Here's how the part is built. I have some questions about the finished solid (model axes, mm). Face numbers are marked on the shaded views. A direction names the side the tool comes from. Coordinates: 2 decimals unless noted, no trailing zeros. Write each loop counter-clockwise with the first axis right and the second up, starting at its lowest first coordinate (ties: lowest second). Pieces come first, ordered by that corner, then holes. Notation, with made-up numbers: (8, 53.25) -> (26, 53.25) arc R9 cw to (26, 63.25) -> close; hole circle Ø9 at (-35, 17.25). An arc over 180 degrees is marked (long way). Use a Markdown table: item, result. Add a question column.
Item 1: Will these pins go through, and if not, where does the flat tip stop? pin 1 Ø4.5 at (y, z) = (-17, -6) entering from -X; pin 2 Ø1.8 at (x, z) = (-5, -5) entering from -Y (3 decimals); pin 3 Ø10 at (y, z) = (-22, 43.5) entering from -X; pin 4 Ø1.9 at (x, z) = (-15.24, -3.81) entering from -Y (3 decimals).
Item 2: If we mould it in two halves opening along X, with no side actions, what happens to the marked faces 1, 2 and 3? For each: pulls with the +X half, pulls with the -X half, needs draft (parallel to the pull), parting line crosses it, or undercut.
Item 3: Imagine slicing it at C-C, the plane x = -21.5. Write out the boundary of the cut face in (y, z) (3 decimals).
Item 4: Imagine slicing it at A-A, the plane z = 13.5. Write out the boundary of the cut face in (x, y) (3 decimals).
Item 5: Imagine slicing it at B-B, the plane x = -10.16. Write out the boundary of the cut face in (y, z) (3 decimals).
Item 6: If I drill on line 1 along Z through (x, y) = (-5, -1) (3 decimals); line 2 along Z through (x, y) = (-13, -2.5) (3 decimals); line 3 along X through (y, z) = (-19, 16) (3 decimals), over which ranges is the centre line in solid material (lowest first)? Write a range as from..to.
Item 7: On a 3-axis mill with a long thin cutter (end or side, diameter ignored), from which of +Z, -Z, +X, -X, +Y, -Y can I reach the whole of each face in a straight line? I mean the marked faces 4, 5, 6, 7 and 8. Say none if no direction works.
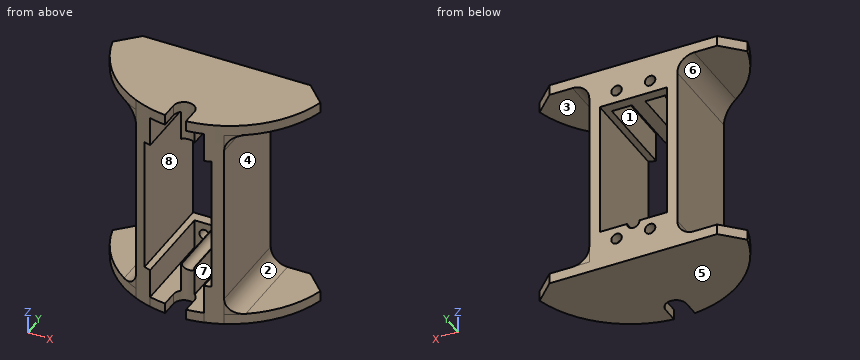
```python
from build123d import *

# Parameters (mm, degrees)
F0_W          = 26.67
F0_H          = 58.928
F0_R          = 1.5875
F1_DEPTH      = 3.175
F2_W          = 4.064
F2_H          = 8.89
F3_DEPTH      = 38.1
F5_DEPTH      = 101.6
F7_DEPTH      = 3.175
F9_DEPTH      = 3.175
F11_DEPTH     = 127
F12_T4_DEPTH  = 40.3062822545
F12_S5_R      = 32.5
F12_T6_DEPTH  = 22
F12_T10_DEPTH = 40.3062822545
F12_S11_R     = 32.5
F12_T12_DEPTH = 22
F12_T16_DEPTH = 40.3062822545
F12_S17_R     = 32.5
F12_T18_DEPTH = 22
F12_T22_DEPTH = 40.3062822545
F12_S23_R     = 32.5
F12_T24_DEPTH = 22


# Not quite as in the source:
# - a fillet or chamfer that OpenCascade refuses, or shapes differently, is made with other operations: its cross-section is extruded or revolved along the edge and cut away or added
# - after a boolean that leaves OpenCascade's solid faulty, fix() repairs it


with BuildPart() as f1:
    # F0 (on Front) → F1 (new body)
    with BuildSketch(Plane.XZ):
        with Locations((-10.16, 20.574)):
            Rectangle(F0_W, F0_H)
        with Locations((-15.24, -3.81)):
            Circle(F0_R, mode=Mode.SUBTRACT)
        with BuildLine():
            Line((0, 41.148), (0, 0))
            Line((0, 0), (-8.255, 0))
            ThreePointArc((-8.255, 0), (-10.16, -1.905), (-12.065, 0))
            Line((-12.065, 0), (-20.32, 0))
            Line((-20.32, 0), (-20.32, 41.148))
            Line((-20.32, 41.148), (0, 41.148))
        make_face(mode=Mode.SUBTRACT)
        with Locations((-5.08, -3.81)):
            Circle(F0_R, mode=Mode.SUBTRACT)
        with Locations((-15.24, 44.958)):
            Circle(F0_R, mode=Mode.SUBTRACT)
        with Locations((-5.08, 44.958)):
            Circle(F0_R, mode=Mode.SUBTRACT)
    extrude(amount=F1_DEPTH)

    # F2 (on face) → F3 (join)
    with BuildSketch(Plane.XZ.offset(3.175)):
        Polygon((0, 0), (-2.032, 0), (-2.032, -8.89), (3.175, -8.89), (3.175, 50.038), (-2.032, 50.038), (-2.032, 41.148), (0, 41.148), align=None)
        with BuildLine():
            Line((-8.128, -8.89), (-8.128, 0))
            Line((-8.128, 0), (-8.255, 0))
            ThreePointArc((-8.255, 0), (-10.16, -1.905), (-12.065, 0))
            Line((-12.065, 0), (-12.192, 0))
            Line((-12.192, 0), (-12.192, -8.89))
            Line((-12.192, -8.89), (-8.128, -8.89))
        make_face()
        Polygon((-23.495, -8.89), (-18.288, -8.89), (-18.288, 0), (-20.32, 0), (-20.32, 41.148), (-18.288, 41.148), (-18.288, 50.038), (-23.495, 50.038), align=None)
        with Locations((-10.16, 45.593)):
            Rectangle(F2_W, F2_H)
    extrude(amount=F3_DEPTH)

    # F4 (on face) → F5 (intersect)
    with BuildSketch(Plane.XY.offset(50.038)):
        with BuildLine():
            Line((-23.495, 0), (-23.495, -27.6062822545))
            ThreePointArc((-23.495, -27.6062822545), (-20.9303918657, -28.6314743475), (-18.288, -29.4352149387))
            Line((-18.288, -29.4352149387), (-18.288, -3.175))
            Line((-18.288, -3.175), (-12.192, -3.175))
            Line((-12.192, -3.175), (-12.192, -30.4044143518))
            ThreePointArc((-12.192, -30.4044143518), (-10.16, -30.468), (-8.128, -30.4044143518))
            Line((-8.128, -30.4044143518), (-8.128, -3.175))
            Line((-8.128, -3.175), (-2.032, -3.175))
            Line((-2.032, -3.175), (-2.032, -29.4352149387))
            ThreePointArc((-2.032, -29.4352149387), (0.6103918657, -28.6314743475), (3.175, -27.6062822545))
            Line((3.175, -27.6062822545), (3.175, 0))
            Line((3.175, 0), (-10.16, 0))
            Line((-10.16, 0), (-23.495, 0))
        make_face()
    extrude(amount=-F5_DEPTH, mode=Mode.INTERSECT)

    # F6 (on face) → F7 (join)
    with BuildSketch(Plane(origin=(0, 0, -8.89), x_dir=(1, 0, 0), z_dir=(0, 0, -1))):
        with BuildLine():
            Line((15.24, 0), (21.313116807, 6.073116807))
            ThreePointArc((21.313116807, 6.073116807), (14.6968126777, 18.9057377838), (3.175, 27.6062822545))
            Line((3.175, 27.6062822545), (3.175, 0))
            Line((3.175, 0), (15.24, 0))
        make_face()
        with BuildLine():
            Line((3.175, 0), (3.175, 27.6062822545))
            ThreePointArc((3.175, 27.6062822545), (0.6103918657, 28.6314743475), (-2.032, 29.4352149387))
            Line((-2.032, 29.4352149387), (-2.032, 3.175))
            Line((-2.032, 3.175), (-8.128, 3.175))
            Line((-8.128, 3.175), (-8.128, 30.4044143518))
            ThreePointArc((-8.128, 30.4044143518), (-10.16, 30.468), (-12.192, 30.4044143518))
            Line((-12.192, 30.4044143518), (-12.192, 3.175))
            Line((-12.192, 3.175), (-18.288, 3.175))
            Line((-18.288, 3.175), (-18.288, 29.4352149387))
            ThreePointArc((-18.288, 29.4352149387), (-20.9303918657, 28.6314743475), (-23.495, 27.6062822545))
            Line((-23.495, 27.6062822545), (-23.495, 0))
            Line((-23.495, 0), (-10.16, 0))
            Line((-10.16, 0), (3.175, 0))
        make_face()
        with BuildLine():
            Line((-2.032, 3.175), (-2.032, 29.4352149387))
            ThreePointArc((-2.032, 29.4352149387), (-5.0569384801, 30.0648653162), (-8.128, 30.4044143518))
            Line((-8.128, 30.4044143518), (-8.128, 3.175))
            Line((-8.128, 3.175), (-2.032, 3.175))
        make_face()
        with BuildLine():
            Line((-12.192, 3.175), (-12.192, 30.4044143518))
            ThreePointArc((-12.192, 30.4044143518), (-15.2630615199, 30.0648653162), (-18.288, 29.4352149387))
            Line((-18.288, 29.4352149387), (-18.288, 3.175))
            Line((-18.288, 3.175), (-12.192, 3.175))
        make_face()
        with BuildLine():
            Line((-35.56, 0), (-23.495, 0))
            Line((-23.495, 0), (-23.495, 27.6062822545))
            ThreePointArc((-23.495, 27.6062822545), (-35.0168126777, 18.9057377838), (-41.633116807, 6.073116807))
            Line((-41.633116807, 6.073116807), (-35.56, 0))
        make_face()
    extrude(amount=F7_DEPTH)

    add(f1.part.fix(), mode=Mode.REPLACE)

    # F8 (on face) → F9 (join)
    with BuildSketch(Plane.XY.offset(50.038)):
        with BuildLine():
            Line((-23.495, -27.6062822545), (-23.495, 0))
            Line((-23.495, 0), (-35.56, 0))
            Line((-35.56, 0), (-41.633116807, -6.073116807))
            ThreePointArc((-41.633116807, -6.073116807), (-35.0168126777, -18.9057377838), (-23.495, -27.6062822545))
        make_face()
        with BuildLine():
            Line((15.24, 0), (3.175, 0))
            Line((3.175, 0), (3.175, -27.6062822545))
            ThreePointArc((3.175, -27.6062822545), (14.6968126777, -18.9057377838), (21.313116807, -6.073116807))
            Line((21.313116807, -6.073116807), (15.24, 0))
        make_face()
        with BuildLine():
            Line((-18.288, -3.175), (-18.288, -29.4352149387))
            ThreePointArc((-18.288, -29.4352149387), (-15.2630615199, -30.0648653162), (-12.192, -30.4044143518))
            Line((-12.192, -30.4044143518), (-12.192, -3.175))
            Line((-12.192, -3.175), (-18.288, -3.175))
        make_face()
        with BuildLine():
            ThreePointArc((-8.128, -30.4044143518), (-5.0569384801, -30.0648653162), (-2.032, -29.4352149387))
            Line((-2.032, -29.4352149387), (-2.032, -3.175))
            Line((-2.032, -3.175), (-8.128, -3.175))
            Line((-8.128, -3.175), (-8.128, -30.4044143518))
        make_face()
        with BuildLine():
            Line((3.175, -27.6062822545), (3.175, 0))
            Line((3.175, 0), (-23.495, 0))
            Line((-23.495, 0), (-23.495, -27.6062822545))
            ThreePointArc((-23.495, -27.6062822545), (-20.9303918657, -28.6314743475), (-18.288, -29.4352149387))
            Line((-18.288, -29.4352149387), (-18.288, -3.175))
            Line((-18.288, -3.175), (-12.192, -3.175))
            Line((-12.192, -3.175), (-12.192, -30.4044143518))
            ThreePointArc((-12.192, -30.4044143518), (-10.16, -30.468), (-8.128, -30.4044143518))
            Line((-8.128, -30.4044143518), (-8.128, -3.175))
            Line((-8.128, -3.175), (-2.032, -3.175))
            Line((-2.032, -3.175), (-2.032, -29.4352149387))
            ThreePointArc((-2.032, -29.4352149387), (0.6103918657, -28.6314743475), (3.175, -27.6062822545))
        make_face()
    extrude(amount=F9_DEPTH)

    # F10 (on face) → F11 (cut)
    with BuildSketch(Plane(origin=(0, 0, -12.065), x_dir=(1, 0, 0), z_dir=(0, 0, -1))):
        with BuildLine():
            Line((-13.335, 30.312541657), (-13.335, 25.4))
            ThreePointArc((-13.335, 25.4), (-10.16, 22.225), (-6.985, 25.4))
            Line((-6.985, 25.4), (-6.985, 30.312541657))
            ThreePointArc((-6.985, 30.312541657), (-10.16, 30.468), (-13.335, 30.312541657))
        make_face()
    extrude(amount=-F11_DEPTH, mode=Mode.SUBTRACT)

    # F12: fillet of radius 5.08 on 4 edges, made by hand


with BuildPart() as f12_tool2:
    # F12_s3 → F12_t4 (new body)
    with BuildSketch(Plane.XZ.offset(40.3062822545)):
        with BuildLine():
            ThreePointArc((-23.495, -3.81), (-24.9828975516, -7.4021024484), (-28.575, -8.89))
            Line((-28.575, -8.89), (-23.495, -8.89))
            Line((-23.495, -8.89), (-23.495, -3.81))
        make_face()
    extrude(amount=-F12_T4_DEPTH)

    # F12_s5 → F12_t6 (intersect, symmetric)
    with BuildSketch(Plane.XY.offset(-6.4)):
        with Locations((-10.16, 2.032)):
            Circle(F12_S5_R)
    extrude(amount=F12_T6_DEPTH, both=True, mode=Mode.INTERSECT)


with BuildPart() as f1_1:
    add(f1.part)

    # F12_t1: union F12_tool2
    add(f12_tool2.part)


with BuildPart() as f12_tool8:
    # F12_s9 → F12_t10 (new body)
    with BuildSketch(Plane.XZ):
        with BuildLine():
            ThreePointArc((-28.575, 50.038), (-24.9828975516, 48.5501024484), (-23.495, 44.958))
            Line((-23.495, 44.958), (-23.495, 50.038))
            Line((-23.495, 50.038), (-28.575, 50.038))
        make_face()
    extrude(amount=F12_T10_DEPTH)

    # F12_s11 → F12_t12 (intersect, symmetric)
    with BuildSketch(Plane.XY.offset(47.5)):
        with Locations((-10.16, 2.032)):
            Circle(F12_S11_R)
    extrude(amount=F12_T12_DEPTH, both=True, mode=Mode.INTERSECT)


with BuildPart() as f1_2:
    add(f1_1.part)

    # F12_t7: union F12_tool8
    add(f12_tool8.part)


with BuildPart() as f12_tool14:
    # F12_s15 → F12_t16 (new body)
    with BuildSketch(Plane.XZ):
        with BuildLine():
            ThreePointArc((3.175, 44.958), (4.6628975516, 48.5501024484), (8.255, 50.038))
            Line((8.255, 50.038), (3.175, 50.038))
            Line((3.175, 50.038), (3.175, 44.958))
        make_face()
    extrude(amount=F12_T16_DEPTH)

    # F12_s17 → F12_t18 (intersect, symmetric)
    with BuildSketch(Plane.XY.offset(47.5)):
        with Locations((-10.16, 2.032)):
            Circle(F12_S17_R)
    extrude(amount=F12_T18_DEPTH, both=True, mode=Mode.INTERSECT)


with BuildPart() as f1_3:
    add(f1_2.part)

    # F12_t13: union F12_tool14
    add(f12_tool14.part)


with BuildPart() as f12_tool20:
    # F12_s21 → F12_t22 (new body)
    with BuildSketch(Plane.XZ.offset(40.3062822545)):
        with BuildLine():
            ThreePointArc((8.255, -8.89), (4.6628975516, -7.4021024484), (3.175, -3.81))
            Line((3.175, -3.81), (3.175, -8.89))
            Line((3.175, -8.89), (8.255, -8.89))
        make_face()
    extrude(amount=-F12_T22_DEPTH)

    # F12_s23 → F12_t24 (intersect, symmetric)
    with BuildSketch(Plane.XY.offset(-6.4)):
        with Locations((-10.16, 2.032)):
            Circle(F12_S23_R)
    extrude(amount=F12_T24_DEPTH, both=True, mode=Mode.INTERSECT)


with BuildPart() as f1_4:
    add(f1_3.part)

    # F12_t19: union F12_tool20
    add(f12_tool20.part)


solid = f1_4.part
```
Ans:
| question | item | result |
|---|---|---|
| 1 | pin 1 | stops at x = -26.11 |
| 1 | pin 2 | stops at y = -3.175 |
| 1 | pin 3 | stops at x = -24.93 |
| 1 | pin 4 | passes through |
| 2 | face 1 | undercut |
| 2 | face 2 | pulls with the +X half |
| 2 | face 3 | needs draft |
| 3 | outline | (-28.425, -12.065) -> (0, -12.065) -> (0, 53.213) -> (-28.425, 53.213) -> close |
| 4 | outline | (-23.495, -27.606) arc R32.5 ccw to (-20.32, -28.839) -> (-20.32, 0) -> (-23.495, 0) -> close; (0, -28.839) arc R32.5 ccw to (3.175, -27.606) -> (3.175, 0) -> (0, 0) -> close |
| 5 | outline | (-22.225, -12.065) -> (0, -12.065) -> (0, -1.905) -> (-22.225, -1.905) -> close; (-22.225, 41.148) -> (0, 41.148) -> (0, 53.213) -> (-22.225, 53.213) -> close |
| 6 | line 1 | z = -12.065..-5.395, -2.225..0, 41.148..43.373, 46.543..53.213 |
| 6 | line 2 | z = -12.065..0, 41.148..53.213 |
| 6 | line 3 | x = -23.495..-20.32, 0..3.175 |
| 7 | face 4 | +X, +Y, -Y |
| 7 | face 5 | -Z, +X, -X, +Y, -Y |
| 7 | face 6 | -X, +Y, -Y |
| 7 | face 7 | -Y |
| 7 | face 8 | +Y, -Y |
